```python
from build123d import *

# Parameters (mm, degrees)
SKETCH_1_R               = 12.5
EXTRUDE_1_DEPTH          = 136
SKETCH_2_R               = 15
EXTRUDE_2_DEPTH          = 70
CHAMFER_1_SIZE           = 1
CUT_EXTRUDE_1_DEPTH      = 4
SKETCH_4_R               = 3
CUT_EXTRUDE_2_DEPTH      = 16
CUT_EXTRUDE_2_DEPTH_BACK = 16


with BuildPart() as part:
    # 草图1 → 凸台-拉伸1 (new body)
    with BuildSketch(Plane(origin=(0, 0, 0), x_dir=(0, 0, -1), z_dir=(1, 0, 0))):
        Circle(SKETCH_1_R)
    extrude(amount=EXTRUDE_1_DEPTH)

    # 草图2 → 凸台-拉伸2 (add)
    with BuildSketch(Plane.ZY):
        Circle(SKETCH_2_R)
    extrude(amount=EXTRUDE_2_DEPTH)

    # 倒角1
    chamfer_1_edges = [part.edges().sort_by_distance(p)[0] for p in [
        (136, 0, 12.5),
        (0, 0, -15),
        (-70, 0, -15),
    ]]
    chamfer(chamfer_1_edges, length=CHAMFER_1_SIZE)

    # 草图3 → 切除-拉伸1 (cut)
    with BuildSketch(Plane.XY.offset(12.5)):
        with BuildLine():
            Line((6, 4), (26, 4))
            ThreePointArc((26, 4), (30, 0), (26, -4))
            Line((26, -4), (6, -4))
            ThreePointArc((6, -4), (2, 0), (6, 4))
        make_face()
        with BuildLine():
            Line((94, 4), (130, 4))
            ThreePointArc((130, 4), (134, 0), (130, -4))
            Line((130, -4), (94, -4))
            ThreePointArc((94, -4), (90, 0), (94, 4))
        make_face()
    extrude(amount=-CUT_EXTRUDE_1_DEPTH, mode=Mode.SUBTRACT)

    # 草图4 → 切除-拉伸2 (cut, two sides)
    with BuildSketch(Plane.XY) as cut_extrude_2_sk:
        with Locations((-30, 0)):
            Circle(SKETCH_4_R)
    extrude(amount=CUT_EXTRUDE_2_DEPTH, mode=Mode.SUBTRACT)
    extrude(cut_extrude_2_sk.sketch, amount=-CUT_EXTRUDE_2_DEPTH_BACK, mode=Mode.SUBTRACT)


solid = part.part
```
Part model, mm, in its own coordinate system. A direction names the side the tool comes from. Round coordinates to 2 decimals unless told otherwise and drop trailing zeros. Loops run counter-clockwise (first coordinate to the right, second up) from the corner with the lowest first, then second, coordinate; pieces in that order, holes last. Notation, with made-up numbers: (83.5, 81) -> (112.5, 81) arc R30 cw to (112.5, 104) -> close; hole circle Ø1 at (-35, 44). An arc over 180 degrees is marked (long way). Use one line per item in the form item = value. Start each with the question number.
Item 1: Band-saw the part on C-C (x = -42.5). List the corners of the cut face in (y, z), plus the area to 3 significant figures.
Item 2: Band-saw the part on A-A (y = 0). List the corners of the cut face in (x, z).
Item 3: Drill centre lines: line 1 along X through (y, z) = (0, -8.75); line 2 along X through (y, z) = (0, 9); line 3 along Y through (x, z) = (123.5, -0.5). Where is each one in solid material? Low to high.
Item 4: Tool access for faces 5 (the flat face through (0, 11.5, -5.3)), 6 (the cylindrical face through (-34.524, 0.66, -14.985)), 7 (the cylindrical face through (134, 0, 11)): list every direction of +Z, -Z, +X, -X, +Y, -Y with a clear straight run to the whole face (end or side of a thin tool).
Item 5: Two-plate mould, pull along Y, no slides. Class faces 1 (the cylindrical face through (66.555, 3.755, -11.923)), 2 (the flat face through (-70, 0, 0)), 3 (the flat face through (16, -4, 10)), 4 (the cylindrical face through (2, 0, 11)): released by +Y, released by -Y, zero draft, split by the parting line, or undercut.
Item 6: Band-saw the part on B-B (x = 34). List the corners of the cut face in (y, z).
Item 7: Drop flat-ended pins along their axis: pin 1 Ø2 at (x, z) = (17.5, -11.5) entering from +Y; pin 2 Ø8 at (x, z) = (99.5, -8) entering from -Y; pin 3 Ø8 at (x, y) = (89, -8) entering from +Z. Give the stop position or say it passes through.
Data:
q1.outline = circle Ø30 at (0, 0)
q1.area = 707 mm^2
q2.outline = (-70, -14) -> (-69, -15) -> (-33, -15) -> (-33, 15) -> (-69, 15) -> (-70, 14) -> close; (-27, -15) -> (-1, -15) -> (0, -14) -> (0, -12.5) -> (135, -12.5) -> (136, -11.5) -> (136, 11.5) -> (135, 12.5) -> (134, 12.5) -> (134, 8.5) -> (90, 8.5) -> (90, 12.5) -> (30, 12.5) -> (30, 8.5) -> (2, 8.5) -> (2, 12.5) -> (0, 12.5) -> (0, 14) -> (-1, 15) -> (-27, 15) -> close
q3.line_1 = -70 to -33, -27 to 136
q3.line_2 = -70 to -33, -27 to 2, 30 to 90, 134 to 136
q3.line_3 = -12.49 to 12.49
q4.face_5 = +X
q4.face_6 = +X, -X
q4.face_7 = +Z
q5.face_1 = split by the parting line
q5.face_2 = zero draft
q5.face_3 = undercut
q5.face_4 = undercut
q6.outline = circle Ø25 at (0, 0)
q7.pin_1 = 6.78
q7.pin_2 = -11.84
q7.pin_3 = 11.84
